Source: CAD feature listing. Evaluate the final solid. Frame: model axes, mm. Face numbers are marked on the shaded views. A direction names the side the tool comes from. Give positions to 0.01 mm unless a question says otherwise; leave off trailing zeros. Write each loop counter-clockwise with the first axis right and the second up, starting at its lowest first coordinate (ties: lowest second). Pieces come first, ordered by that corner, then holes. Notation, with made-up numbers: M 59,76.5 L 74,76.5 A32 cw 74,106.5 Z; hole C 28,43.25 d9. An arc over 180 degrees is marked long. Use CSV: the item, a comma, the result in double quotes. Start each with the question number.
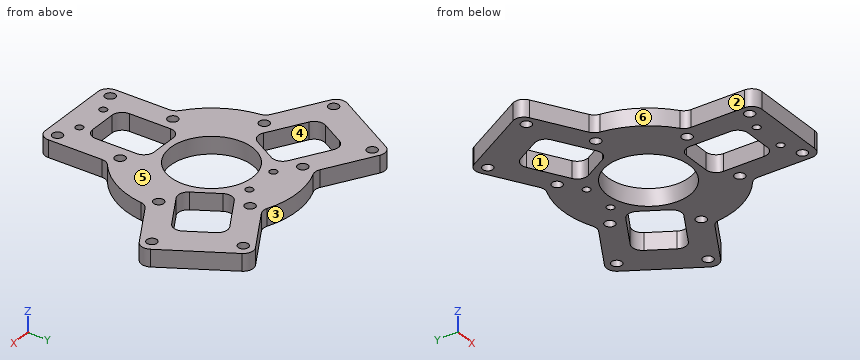
from build123d import *

# Parameters (mm, degrees)
SKETCH1_R           = 25
BOSS_EXTRUDE1_DEPTH = 5
CUT_EXTRUDE1_REACH  = 61.269
SKETCH2_R           = 1.5
FILLET1_R           = 3
CUT_EXTRUDE2_REACH  = 60.487
SKETCH3_R           = 1.1
CUT_EXTRUDE3_REACH  = 60.487
SKETCH4_R           = 1.5
FILLET2_R           = 3
CUT_EXTRUDE4_REACH  = 60.487
SKETCH5_R           = 12
SKETCH5_W           = 14
SKETCH5_H           = 18
FILLET3_R           = 3


with BuildPart() as part:
    # Sketch1 → Boss-Extrude1 (new body)
    with BuildSketch(Plane.XY):
        with BuildLine():
            ThreePointArc((-24.937391115, -1.768198064), (-21.650635095, 12.5), (-10.937391115, 22.480513242))
            Line((-10.937391115, 22.480513242), (-28.507041555, 32.624355653))
            Line((-28.507041555, 32.624355653), (-42.507041555, 8.375644347))
            Line((-42.507041555, 8.375644347), (-24.937391115, -1.768198064))
        make_face()
        Circle(SKETCH1_R)
        with BuildLine():
            Line((28.507041555, 32.624355653), (10.937391115, 22.480513242))
            ThreePointArc((10.937391115, 22.480513242), (21.194749089, 13.258303476), (25, 0))
            ThreePointArc((25, 0), (24.984342876, -0.884653077), (24.937391115, -1.768198064))
            Line((24.937391115, -1.768198064), (42.507041555, 8.375644347))
            Line((42.507041555, 8.375644347), (28.507041555, 32.624355653))
        make_face()
        with BuildLine():
            ThreePointArc((14, -20.712315177), (0, -25), (-14, -20.712315177))
            Line((-14, -20.712315177), (-14, -41))
            Line((-14, -41), (14, -41))
            Line((14, -41), (14, -20.712315177))
        make_face()
    extrude(amount=BOSS_EXTRUDE1_DEPTH)

    # Sketch2 → Cut-Extrude1 (cut, up to next)
    with BuildSketch(Plane.XY.offset(5), mode=Mode.PRIVATE) as cut_extrude1_sk1:
        with Locations((11, -37.4)):
            Circle(SKETCH2_R)
    cut_extrude1_tool1 = extrude(cut_extrude1_sk1.sketch, amount=-CUT_EXTRUDE1_REACH, mode=Mode.PRIVATE) & part.part
    # Sketch2 → Cut-Extrude1 (cut, up to next)
    with BuildSketch(Plane.XY.offset(5), mode=Mode.PRIVATE) as cut_extrude1_sk2:
        with Locations((-11, -37.4)):
            Circle(SKETCH2_R)
    cut_extrude1_tool2 = extrude(cut_extrude1_sk2.sketch, amount=-CUT_EXTRUDE1_REACH, mode=Mode.PRIVATE) & part.part
    # Sketch2 → Cut-Extrude1 (cut, up to next)
    with BuildSketch(Plane.XY.offset(5), mode=Mode.PRIVATE) as cut_extrude1_sk3:
        with Locations((-37.889350102, 9.173720558)):
            Circle(SKETCH2_R)
    cut_extrude1_tool3 = extrude(cut_extrude1_sk3.sketch, amount=-CUT_EXTRUDE1_REACH, mode=Mode.PRIVATE) & part.part
    # Sketch2 → Cut-Extrude1 (cut, up to next)
    with BuildSketch(Plane.XY.offset(5), mode=Mode.PRIVATE) as cut_extrude1_sk4:
        with Locations((-26.889350102, 28.226279442)):
            Circle(SKETCH2_R)
    cut_extrude1_tool4 = extrude(cut_extrude1_sk4.sketch, amount=-CUT_EXTRUDE1_REACH, mode=Mode.PRIVATE) & part.part
    # Sketch2 → Cut-Extrude1 (cut, up to next)
    with BuildSketch(Plane.XY.offset(5), mode=Mode.PRIVATE) as cut_extrude1_sk5:
        with Locations((26.889350102, 28.226279442)):
            Circle(SKETCH2_R)
    cut_extrude1_tool5 = extrude(cut_extrude1_sk5.sketch, amount=-CUT_EXTRUDE1_REACH, mode=Mode.PRIVATE) & part.part
    # Sketch2 → Cut-Extrude1 (cut, up to next)
    with BuildSketch(Plane.XY.offset(5), mode=Mode.PRIVATE) as cut_extrude1_sk6:
        with Locations((37.889350102, 9.173720558)):
            Circle(SKETCH2_R)
    cut_extrude1_tool6 = extrude(cut_extrude1_sk6.sketch, amount=-CUT_EXTRUDE1_REACH, mode=Mode.PRIVATE) & part.part
    add(cut_extrude1_tool1.solids().sort_by_distance((11, -37.4, 5))[0], mode=Mode.SUBTRACT)
    add(cut_extrude1_tool2.solids().sort_by_distance((-11, -37.4, 5))[0], mode=Mode.SUBTRACT)
    add(cut_extrude1_tool3.solids().sort_by_distance((-37.88935, 9.173721, 5))[0], mode=Mode.SUBTRACT)
    add(cut_extrude1_tool4.solids().sort_by_distance((-26.88935, 28.226279, 5))[0], mode=Mode.SUBTRACT)
    add(cut_extrude1_tool5.solids().sort_by_distance((26.88935, 28.226279, 5))[0], mode=Mode.SUBTRACT)
    add(cut_extrude1_tool6.solids().sort_by_distance((37.88935, 9.173721, 5))[0], mode=Mode.SUBTRACT)

    # Fillet1
    fillet1_edges = [part.edges().sort_by_distance(p)[0] for p in [
        (-42.507041555, 8.375644347, 2.5),
        (-28.507041555, 32.624355653, 2.5),
        (28.507041555, 32.624355653, 2.5),
        (42.507041555, 8.375644347, 2.5),
        (14, -41, 2.5),
        (-14, -41, 2.5),
    ]]
    fillet(fillet1_edges, radius=FILLET1_R)

    # Sketch3 → Cut-Extrude2 (cut, up to next)
    with BuildSketch(Plane(origin=(0, 0, 0), x_dir=(-1, 0, 0), z_dir=(0, 0, -1)), mode=Mode.PRIVATE) as cut_extrude2_sk1:
        with Locations((5.030631655, 14.595653448)):
            Circle(SKETCH3_R)
    cut_extrude2_tool1 = extrude(cut_extrude2_sk1.sketch, amount=-CUT_EXTRUDE2_REACH, mode=Mode.PRIVATE) & part.part
    # Sketch3 → Cut-Extrude2 (cut, up to next)
    with BuildSketch(Plane(origin=(0, 0, 0), x_dir=(-1, 0, 0), z_dir=(0, 0, -1)), mode=Mode.PRIVATE) as cut_extrude2_sk2:
        with Locations((-4.969346288, 14.61665653)):
            Circle(SKETCH3_R)
    cut_extrude2_tool2 = extrude(cut_extrude2_sk2.sketch, amount=-CUT_EXTRUDE2_REACH, mode=Mode.PRIVATE) & part.part
    # Sketch3 → Cut-Extrude2 (cut, up to next)
    with BuildSketch(Plane(origin=(0, 0, 0), x_dir=(-1, 0, 0), z_dir=(0, 0, -1)), mode=Mode.PRIVATE) as cut_extrude2_sk3:
        with Locations((4.926079941, -35.183463358)):
            Circle(SKETCH3_R)
    cut_extrude2_tool3 = extrude(cut_extrude2_sk3.sketch, amount=-CUT_EXTRUDE2_REACH, mode=Mode.PRIVATE) & part.part
    # Sketch3 → Cut-Extrude2 (cut, up to next)
    with BuildSketch(Plane(origin=(0, 0, 0), x_dir=(-1, 0, 0), z_dir=(0, 0, -1)), mode=Mode.PRIVATE) as cut_extrude2_sk4:
        with Locations((-5.073898003, -35.162460277)):
            Circle(SKETCH3_R)
    cut_extrude2_tool4 = extrude(cut_extrude2_sk4.sketch, amount=-CUT_EXTRUDE2_REACH, mode=Mode.PRIVATE) & part.part
    add(cut_extrude2_tool1.solids().sort_by_distance((-5.030632, 14.595653, 0))[0], mode=Mode.SUBTRACT)
    add(cut_extrude2_tool2.solids().sort_by_distance((4.969346, 14.616657, 0))[0], mode=Mode.SUBTRACT)
    add(cut_extrude2_tool3.solids().sort_by_distance((-4.92608, -35.183463, 0))[0], mode=Mode.SUBTRACT)
    add(cut_extrude2_tool4.solids().sort_by_distance((5.073898, -35.16246, 0))[0], mode=Mode.SUBTRACT)

    # Sketch4 → Cut-Extrude3 (cut, up to next)
    with BuildSketch(Plane.XY.offset(5), mode=Mode.PRIVATE) as cut_extrude3_sk1:
        with Locations((22, 0)):
            Circle(SKETCH4_R)
    cut_extrude3_tool1 = extrude(cut_extrude3_sk1.sketch, amount=-CUT_EXTRUDE3_REACH, mode=Mode.PRIVATE) & part.part
    # Sketch4 → Cut-Extrude3 (cut, up to next)
    with BuildSketch(Plane.XY.offset(5), mode=Mode.PRIVATE) as cut_extrude3_sk2:
        with Locations((11, -19.052558883)):
            Circle(SKETCH4_R)
    cut_extrude3_tool2 = extrude(cut_extrude3_sk2.sketch, amount=-CUT_EXTRUDE3_REACH, mode=Mode.PRIVATE) & part.part
    # Sketch4 → Cut-Extrude3 (cut, up to next)
    with BuildSketch(Plane.XY.offset(5), mode=Mode.PRIVATE) as cut_extrude3_sk3:
        with Locations((-11, -19.052558883)):
            Circle(SKETCH4_R)
    cut_extrude3_tool3 = extrude(cut_extrude3_sk3.sketch, amount=-CUT_EXTRUDE3_REACH, mode=Mode.PRIVATE) & part.part
    # Sketch4 → Cut-Extrude3 (cut, up to next)
    with BuildSketch(Plane.XY.offset(5), mode=Mode.PRIVATE) as cut_extrude3_sk4:
        with Locations((-22, 0)):
            Circle(SKETCH4_R)
    cut_extrude3_tool4 = extrude(cut_extrude3_sk4.sketch, amount=-CUT_EXTRUDE3_REACH, mode=Mode.PRIVATE) & part.part
    # Sketch4 → Cut-Extrude3 (cut, up to next)
    with BuildSketch(Plane.XY.offset(5), mode=Mode.PRIVATE) as cut_extrude3_sk5:
        with Locations((-11, 19.052558883)):
            Circle(SKETCH4_R)
    cut_extrude3_tool5 = extrude(cut_extrude3_sk5.sketch, amount=-CUT_EXTRUDE3_REACH, mode=Mode.PRIVATE) & part.part
    # Sketch4 → Cut-Extrude3 (cut, up to next)
    with BuildSketch(Plane.XY.offset(5), mode=Mode.PRIVATE) as cut_extrude3_sk6:
        with Locations((11, 19.052558883)):
            Circle(SKETCH4_R)
    cut_extrude3_tool6 = extrude(cut_extrude3_sk6.sketch, amount=-CUT_EXTRUDE3_REACH, mode=Mode.PRIVATE) & part.part
    add(cut_extrude3_tool1.solids().sort_by_distance((22, 0, 5))[0], mode=Mode.SUBTRACT)
    add(cut_extrude3_tool2.solids().sort_by_distance((11, -19.052559, 5))[0], mode=Mode.SUBTRACT)
    add(cut_extrude3_tool3.solids().sort_by_distance((-11, -19.052559, 5))[0], mode=Mode.SUBTRACT)
    add(cut_extrude3_tool4.solids().sort_by_distance((-22, 0, 5))[0], mode=Mode.SUBTRACT)
    add(cut_extrude3_tool5.solids().sort_by_distance((-11, 19.052559, 5))[0], mode=Mode.SUBTRACT)
    add(cut_extrude3_tool6.solids().sort_by_distance((11, 19.052559, 5))[0], mode=Mode.SUBTRACT)

    # Fillet2
    fillet2_edges = [part.edges().sort_by_distance(p)[0] for p in [
        (-10.937391115, 22.480513242, 2.5),
        (10.937391115, 22.480513242, 2.5),
        (24.937391115, -1.768198064, 2.5),
        (14, -20.712315177, 2.5),
        (-14, -20.712315177, 2.5),
        (-24.937391115, -1.768198064, 2.5),
    ]]
    fillet(fillet2_edges, radius=FILLET2_R)

    # Sketch5 → Cut-Extrude4 (cut, up to next)
    with BuildSketch(Plane.XY.offset(5), mode=Mode.PRIVATE) as cut_extrude4_sk1:
        Circle(SKETCH5_R)
    cut_extrude4_tool1 = extrude(cut_extrude4_sk1.sketch, amount=-CUT_EXTRUDE4_REACH, mode=Mode.PRIVATE) & part.part
    # Sketch5 → Cut-Extrude4 (cut, up to next)
    with BuildSketch(Plane.XY.offset(5), mode=Mode.PRIVATE) as cut_extrude4_sk2:
        Polygon((-8.624355653, 13.062177826), (-15.624355653, 0.937822174), (-31.212812921, 9.937822174), (-24.212812921, 22.062177826), align=None)
    cut_extrude4_tool2 = extrude(cut_extrude4_sk2.sketch, amount=-CUT_EXTRUDE4_REACH, mode=Mode.PRIVATE) & part.part
    # Sketch5 → Cut-Extrude4 (cut, up to next)
    with BuildSketch(Plane.XY.offset(5), mode=Mode.PRIVATE) as cut_extrude4_sk3:
        with Locations((0, -23)):
            Rectangle(SKETCH5_W, SKETCH5_H)
    cut_extrude4_tool3 = extrude(cut_extrude4_sk3.sketch, amount=-CUT_EXTRUDE4_REACH, mode=Mode.PRIVATE) & part.part
    # Sketch5 → Cut-Extrude4 (cut, up to next)
    with BuildSketch(Plane.XY.offset(5), mode=Mode.PRIVATE) as cut_extrude4_sk4:
        Polygon((15.624355653, 0.937822174), (8.624355653, 13.062177826), (24.212812921, 22.062177826), (31.212812921, 9.937822174), align=None)
    cut_extrude4_tool4 = extrude(cut_extrude4_sk4.sketch, amount=-CUT_EXTRUDE4_REACH, mode=Mode.PRIVATE) & part.part
    add(cut_extrude4_tool1.solids().sort_by_distance((0, 0, 5))[0], mode=Mode.SUBTRACT)
    add(cut_extrude4_tool2.solids().sort_by_distance((-19.918584, 11.5, 5))[0], mode=Mode.SUBTRACT)
    add(cut_extrude4_tool3.solids().sort_by_distance((0, -23, 5))[0], mode=Mode.SUBTRACT)
    add(cut_extrude4_tool4.solids().sort_by_distance((19.918584, 11.5, 5))[0], mode=Mode.SUBTRACT)

    # Fillet3
    fillet3_edges = [part.edges().sort_by_distance(p)[0] for p in [
        (8.624355653, 13.062177826, 2.5),
        (24.212812921, 22.062177826, 2.5),
        (31.212812921, 9.937822174, 2.5),
        (15.624355653, 0.937822174, 2.5),
        (-15.624355653, 0.937822174, 2.5),
        (-31.212812921, 9.937822174, 2.5),
        (-24.212812921, 22.062177826, 2.5),
        (-8.624355653, 13.062177826, 2.5),
        (7, -14, 2.5),
        (7, -32, 2.5),
        (-7, -32, 2.5),
        (-7, -14, 2.5),
    ]]
    fillet(fillet3_edges, radius=FILLET3_R)


solid = part.part
1. Line query: probe 1 along Y at (x, z) = (-2, 3.9); probe 2 along X at (y, z) = (28, 0.5); probe 3 along X at (y, z) = (8, 2.8). Output: solid intervals per line, ascending.
2. Section C-C on x = 33.5. Return loops of the section in (y, z), then the cut area to 3 significant figures.
3. Section D-D on y = -13. Return loops of the section in (x, z), then the cut area to 3 significant figures.
4. Section B-B on y = 0. Return loops of the section in (x, z), then the cut area to 3 significant figures.
5. Access query for the marked faces 1, 2 and 3. Directions: +Z, -Z, +X, -X, +Y, -Y. A direction counts if a zero-diameter tool reaches every point of the face in a straight line with its end or side. Return the directions, or none.
6. First-contact query: pin 1 (1.5 mm diameter, centred on x = 32.5, z = 2, fed in from +Y); pin 2 (2.5 mm diameter, centred on x = 11, y = -37.4, fed in from +Z); pin 3 (2.5 mm diameter, centred on y = -25.5, z = 2, fed in from +X). Flat tips, straight axial feed; report the tip coordinate or a pass-through.
7. Pull-direction query (X, two-part tool) for the marked faces 4, 5 and 6; classes: released by +X, released by -X, zero draft, split by the parting line, or undercut.
8. Section A-A on x = 0. Return loops of the section in (y, z), then the cut area to 3 significant figures.
Resolved:
1,probe 1,"y = -41 to -32, -14 to -11.83, 11.83 to 24.92"
1,probe 2,"x = -31.18 to -28.37, -25.41 to -20.5, 20.5 to 25.41, 28.37 to 31.18"
1,probe 3,"x = -41.02 to -38.82, -36.96 to -27.86, -11.55 to -8.94, 8.94 to 11.55, 27.86 to 36.96, 38.82 to 41.02"
2,outline,"M 3.18,0 L 23.98,0 L 23.98,5 L 3.18,5 Z"
2,area,"104 mm2"
3,outline,"M -21.35,0 L 21.35,0 L 21.35,5 L -21.35,5 Z"
3,area,"214 mm2"
4,outline,"M -28,0 L -23.5,0 L -23.5,5 L -28,5 Z; M -20.5,0 L -12,0 L -12,5 L -20.5,5 Z; M 12,0 L 20.5,0 L 20.5,5 L 12,5 Z; M 23.5,0 L 28,0 L 28,5 L 23.5,5 Z"
4,area,"130 mm2"
5,face 1,"+Z, -Z"
5,face 2,"+Z, -Z, -X, -Y"
5,face 3,"+Z, -Z, +Y"
6,pin 1,"stops at y = 27.01"
6,pin 2,"passes through"
6,pin 3,"stops at x = 14"
7,face 4,"undercut"
7,face 5,"zero draft"
7,face 6,"released by -X"
8,outline,"M -41,0 L -32,0 L -32,5 L -41,5 Z; M -14,0 L -12,0 L -12,5 L -14,5 Z; M 12,0 L 25,0 L 25,5 L 12,5 Z"
8,area,"120 mm2"
